```python
from build123d import *

# Parameters (mm, degrees)
SKETCH1_W                      = 50.8
SKETCH1_H                      = 9.525
BOSS_EXTRUDE1_DEPTH            = 38.1
F_5_16_0_3125_DIAMETER_HOLE1_D = 7.9375
F_8_32_TAPPED_HOLE1_D          = 3.4544
F_8_32_TAPPED_HOLE1_DEPTH      = 25.4
F_8_32_TAPPED_HOLE1_TIP        = 1.037806461


with BuildPart() as part:
    # Sketch1 → Boss-Extrude1 (new body)
    with BuildSketch(Plane.XY):
        Rectangle(SKETCH1_W, SKETCH1_H)
    extrude(amount=BOSS_EXTRUDE1_DEPTH)

    # 5/16 (0.3125) Diameter Hole1 (through all)
    with Locations(Plane(origin=(0, -4.7625, 0), x_dir=(-1, 0, 0), z_dir=(0, -1, 0))):
        with Locations((0, -12.7), (0, -27.94)):
            Hole(F_5_16_0_3125_DIAMETER_HOLE1_D / 2)

    # #8-32 Tapped Hole1
    with Locations(Plane(origin=(0, 0, 0), x_dir=(-1, 0, 0), z_dir=(0, 0, -1))):
        with Locations((-12.7, 0), (12.7, 0)):
            Hole(F_8_32_TAPPED_HOLE1_D / 2, depth=F_8_32_TAPPED_HOLE1_DEPTH)
            with Locations((0, 0, -(F_8_32_TAPPED_HOLE1_DEPTH + F_8_32_TAPPED_HOLE1_TIP / 2))):  # 118° drill point
                Cone(0, F_8_32_TAPPED_HOLE1_D / 2, F_8_32_TAPPED_HOLE1_TIP, mode=Mode.SUBTRACT)


solid = part.part
```
CAD build for the part. Positions are in the model's coordinates, mm. A direction names the side the tool comes from. Coordinates: 2 decimals unless noted, no trailing zeros. Write each loop counter-clockwise with the first axis right and the second up, starting at its lowest first coordinate (ties: lowest second). Pieces come first, ordered by that corner, then holes. Notation, with made-up numbers: (44, -24) -> (96, -24) arc R10 cw to (96, -8) -> close; hole circle Ø8 at (53.5, 74.25). An arc over 180 degrees is marked (long way). Return JSON: item names as keys, results as strings. Group by question number.
Q1. Pull direction X, two halves, no side cores. Call faces 1 (the face through (-0.517, 0.067, 24.005)), 2 (the face through (25.4, 0, 19)), 3 (the face through (0, -4.762, 19)): released by +X, released by -X, zero draft, split by the parting line, or undercut.
Q2. Flat gauge pin, fed straight in: pin 1 (9 mm diameter, centred on x = 0, z = 27.94, fed in from -Y). Where does the tip first touch, or does it go through?
Q3. Cut at A-A, the plane z = 12.7. Give the cut face in (x, y), then the cut area to 3 significant figures.
Q4. Cut at B-B, the plane x = 0. Give the cut face in (y, z).
Q5. Cut at D-D, the plane z = 27.94. Give the cut face in (x, y), then the cut area to 3 significant figures.
Q6. Which spindle directions (+Z, -Z, +X, -X, +Y, -Y) get a long thin tool onto all of the face, cutting with end or side? Do faces 4 (the face through (14.295, -0.662, 12.878)), 5 (the face through (0, 4.762, 19)). Say none if no direction does.
Q7. Cut at C-C, the plane y = -3.75. Give the cut face in (x, z), then the cut area to 3 significant figures.
Q8. Drill centre lines: line 1 (X direction, y = 0, z = 18.25); line 2 (Z direction, x = 0, y = -0.25); line 3 (Z direction, x = -3, y = -0.5). Where is each one in solid material? Low to high.
Returned:
{
 "1": {"face 1": "undercut", "face 2": "released by +X", "face 3": "zero draft"},
 "2": {"pin 1": "stops at y = -4.76"},
 "3": {"outline": "(-25.4, -4.76) -> (-3.97, -4.76) -> (-3.97, 4.76) -> (-25.4, 4.76) -> close; (3.97, -4.76) -> (25.4, -4.76) -> (25.4, 4.76) -> (3.97, 4.76) -> close; hole circle Ø3.45 at (-12.7, 0); hole circle Ø3.45 at (12.7, 0)", "area": "390 mm2"},
 "4": {"outline": "(-4.76, 0) -> (4.76, 0) -> (4.76, 8.73) -> (-4.76, 8.73) -> close; (-4.76, 16.67) -> (4.76, 16.67) -> (4.76, 23.97) -> (-4.76, 23.97) -> close; (-4.76, 31.91) -> (4.76, 31.91) -> (4.76, 38.1) -> (-4.76, 38.1) -> close"},
 "5": {"outline": "(-25.4, -4.76) -> (-3.97, -4.76) -> (-3.97, 4.76) -> (-25.4, 4.76) -> close; (3.97, -4.76) -> (25.4, -4.76) -> (25.4, 4.76) -> (3.97, 4.76) -> close", "area": "408 mm2"},
 "6": {"face 4": "-Z", "face 5": "+Z, -Z, +X, -X, +Y"},
 "7": {"outline": "(-25.4, 0) -> (25.4, 0) -> (25.4, 38.1) -> (-25.4, 38.1) -> close; hole circle Ø7.94 at (0, 12.7); hole circle Ø7.94 at (0, 27.94)", "area": "1,840 mm2"},
 "8": {"line 1": "x = -25.4 to -14.43, -10.97 to 10.97, 14.43 to 25.4", "line 2": "z = 0 to 8.73, 16.67 to 23.97, 31.91 to 38.1", "line 3": "z = 0 to 10.1, 15.3 to 25.34, 30.54 to 38.1"}
}
